Work out the finished part from the listing and answer in its coordinate system (mm). A direction names the side the tool comes from. Give positions to 0.01 mm unless a question says otherwise; leave off trailing zeros. Order: outer loops, then holes, each group sorted by start corner. A loop starts at its lowest first (then second) coordinate and runs counter-clockwise, first axis right, second up.
Autodesk Inventor part; units mm, degrees
sketch "Sketch1" plane through (0, 0, 0) normal (0, 0, 1) x (1, 0, 0)
  line L0 (-4.55, 7.5) -> (4.55, 7.5)
  line L1 (4.55, 7.5) -> (4.55, -7.5)
  line L2 (4.55, -7.5) -> (-4.55, -7.5)
  line L3 (-4.55, -7.5) -> (-4.55, 7.5)
  line L4 (-4.55, 7.5) -> (4.55, -7.5) construction
  line L5 (4.55, 7.5) -> (-4.55, -7.5) construction
  line L6 (-2.05, -2.05) -> (2.05, -2.05)
  line L7 (2.05, -2.05) -> (2.05, 2.05)
  line L8 (2.05, 2.05) -> (-2.05, 2.05)
  line L9 (-2.05, 2.05) -> (-2.05, -2.05)
  line L10 (-2.05, -2.05) -> (2.05, 2.05) construction
  line L11 (2.05, -2.05) -> (-2.05, 2.05) construction
  line L12 (-4.55, 7.5) -> (-16.55, 7.5)
  line L13 (-16.55, 7.5) -> (-16.55, 6)
  line L14 (-16.55, 6) -> (-4.55, 6)
  line L15 (-4.55, 6) -> (-4.55, 7.5)
  line L16 (-4.55, -7.5) -> (-16.55, -7.5)
  line L17 (-16.55, -7.5) -> (-16.55, -6)
  line L18 (-16.55, -6) -> (-4.55, -6)
  line L19 (-4.55, -6) -> (-4.55, -7.5)
  line L20 (4.55, 7.5) -> (16.55, 7.5)
  line L21 (16.55, 7.5) -> (16.55, 6)
  line L22 (16.55, 6) -> (4.55, 6)
  line L23 (4.55, 6) -> (4.55, 7.5)
  line L24 (4.55, -7.5) -> (16.55, -7.5)
  line L25 (16.55, -7.5) -> (16.55, -6)
  line L26 (16.55, -6) -> (4.55, -6)
  line L27 (4.55, -6) -> (4.55, -7.5)
  point P0 (0, 0)
  point P1 (-4.55, 6)
  point P2 (-4.55, -6)
  point P3 (4.55, 6)
  dimension "d0" = 15
  dimension "d1" = 9.1
  dimension "d2" = 4.1
  dimension "d3" = 4.1
  dimension "d4" = 12
  dimension "d5" = 1.5
  dimension "d8" = 1.5
  dimension "d9" = 12
  dimension "d10" = 12
  dimension "d11" = 1.5
  dimension "d12" = 12
extrude "Extrusion1" add sketch "Sketch1" along normal blind 12
sketch "Sketch2" plane through (0, 0, 12) normal (0, 0, 1) x (1, 0, 0)
  line L0 (16.55, 7.5) -> (-16.55, 7.5)
  line L1 (-3.7, 7.5) -> (-1.7, 7.5)
  line L2 (-1.7, 7.5) -> (-1.7, 14.5)
  line L3 (-1.7, 14.5) -> (-3.7, 14.5)
  line L4 (-3.7, 14.5) -> (-3.7, 7.5)
  line L5 (1.7, 7.5) -> (3.7, 7.5)
  line L6 (3.7, 7.5) -> (3.7, 14.5)
  line L7 (3.7, 14.5) -> (1.7, 14.5)
  line L8 (1.7, 14.5) -> (1.7, 7.5)
  point P0 (0, 0)
  dimension "d15" = 2
  dimension "d16" = 2
  dimension "d17" = 7
  dimension "d18" = 7
  dimension "d19" = 1.7
  dimension "d20" = 1.7
extrude "Extrusion2" add sketch "Sketch2" against normal up to surface (12 mm away)
fillet "Fillet1" radius 8 2 edges at (3.7, 7.5, 6) (-3.7, 7.5, 6)
sketch "Sketch3" plane through (4.55, -6, 0) normal (1, 0, 0) x (0, 0, -1)
  line L0 (-6.4, 3.1) -> (-5.6, 3.1)
  line L1 (-5.6, 3.1) -> (-5.6, 0)
  line L2 (-5.6, 0) -> (-6.4, 0)
  line L3 (-6.4, 0) -> (-6.4, 3.1)
  line L4 (0, 12) -> (-12, 12)
  line L5 (0, 0) -> (0, 12)
  line L6 (0, 0) -> (-12, 0)
  point P0 (0, 6)
  dimension "d24" = 3.1
  dimension "d25" = 0.8
  dimension "d30" = 0
  dimension "d39" = 12
  dimension "d40" = 5.6
extrude "Extrusion3" cut sketch "Sketch3" against normal through all
sketch "Sketch5" plane through (0, 0, 0) normal (0, 0, -1) x (-1, 0, 0)
  line L0 (-2.05, 5.05) -> (2.05, 5.05)
  line L1 (2.05, 5.05) -> (2.05, 3.55)
  line L2 (2.05, 3.55) -> (-2.05, 3.55)
  line L3 (-2.05, 3.55) -> (-2.05, 5.05)
  line L4 (-2.05, -3.55) -> (2.05, -3.55)
  line L5 (2.05, -3.55) -> (2.05, -5.05)
  line L6 (2.05, -5.05) -> (-2.05, -5.05)
  line L7 (-2.05, -5.05) -> (-2.05, -3.55)
  line L8 (2.05, 2.05) -> (-2.05, 2.05)
  line L9 (2.05, -2.05) -> (2.05, 2.05)
  line L10 (-2.05, -2.05) -> (2.05, -2.05)
  point P0 (0, 0)
  dimension "d31" = 4.1
  dimension "d32" = 4.1
  dimension "d33" = 1.5
  dimension "d34" = 1.5
  dimension "d35" = 1.5
  dimension "d36" = 1.5
extrude "Extrusion4" cut sketch "Sketch5" against normal through all
fillet "Fillet2" radius 2 8 edges at (-16.55, 6.75, 0) (-16.55, 6.75, 12) (-16.55, -6.75, 0) (-16.55, -6.75, 12) (16.55, 6.75, 12) (16.55, -6.75, 12) (16.55, 6.75, 0) (16.55, -6.75, 0)
equation "\"d40\" = -0.5 * d25 + 0.5 * d39"
equation "\"d31\" = d32"
properties part number "wing_honeycomb_interface"
1. Which of the six approach directions +Z, -Z, +X, -X, +Y, -Y give full straight-line access (tool end or side, diameter ignored) to faces 4 (the face through (-4.55, 0, 6)), 5 (the face through (0, 3.55, 6)), 6 (the face through (4.55, 0, 6))?
Findings below:
face 4: +Z, -Z, -X
face 5: +Z, -Z
face 6: +Z, -Z, +X
2. The mould has two halves that part along Y. Classify faces 1 (the face through (15.95, -6.74, 11.43)), 2 (the face through (6.29, 9.55, 6.08)), 3 (the face through (-2.05, -4, 3)): pulls with the +Y half, pulls with the -Y half, needs draft (parallel to the pull), parting line crosses it, or undercut.
Findings below:
face 1: needs draft
face 2: pulls with the +Y half
face 3: undercut
3. The part is cut by section C-C (y = -1.25). Write down the section's boundary in (x, z), then the cut area to 3 significant figures.
Findings below:
outline: (-4.55, 0) - (-2.05, 0) - (-2.05, 12) - (-4.55, 12) - close; (2.05, 0) - (4.55, 0) - (4.55, 12) - (2.05, 12) - close
area: 60.0 mm2
4. Given P1, Ø4, axis at y = -1, z = 8.5, coming from the -X side; P2, Ø2, axis at y = 0, z = 5.5, coming from the +X side; P3, Ø4.5, axis at x = 0, z = 2, coming from the +Y side; P4, Ø2, axis at y = 12, z = 8, coming from the +X side, each flat-ended and moving along its own axis, determine where each tip first touches the part or whether it passes through.
Findings below:
P1: stops at x = -4.55
P2: stops at x = 4.55
P3: stops at y = 14.5
P4: stops at x = 5.02
5. Straight lines are drawn through the part: probe 1 along Y at (x, z) = (2, 9); probe 2 along Y at (x, z) = (14, 3.75); probe 3 along X at (y, z) = (-1.25, 9). For each, find the intervals that lie inside material, in ascending order.
Findings below:
probe 1: y = -7.5 to -5.05, -3.55 to -2.05, 2.05 to 3.55, 5.05 to 14.5
probe 2: y = -7.5 to -6, 6 to 7.5
probe 3: x = -4.55 to -2.05, 2.05 to 4.55
6. The part is cut by section A-A (y = -4.5). Write down the section's boundary in (x, z).
Findings below:
outline: (-4.55, 0) - (-2.05, 0) - (-2.05, 5.6) - (-4.55, 5.6) - close; (-4.55, 6.4) - (-2.05, 6.4) - (-2.05, 12) - (-4.55, 12) - close; (2.05, 0) - (4.55, 0) - (4.55, 5.6) - (2.05, 5.6) - close; (2.05, 6.4) - (4.55, 6.4) - (4.55, 12) - (2.05, 12) - close
7. The part is cut by section B-B (x = -9). Write down the section's boundary in (y, z), then the cut area to 3 significant figures.
Findings below:
outline: (-7.5, 0) - (-6, 0) - (-6, 12) - (-7.5, 12) - close; (6, 0) - (7.95, 0) - (7.95, 12) - (6, 12) - close
area: 41.4 mm2
8. The part is cut by section D-D (z = 8.75). State how many separate pieces and enclosed holes the cut face has, then the cut area to 3 significant figures.
Findings below:
separate pieces: 1
enclosed holes: 3
area: 234 mm2
